Autodesk Inventor part; units mm, degrees
ref_plane "YZ Plane" through (0, 0, 0) normal (1, 0, 0) x (0, 1, 0)
ref_plane "XZ Plane" through (0, 0, 0) normal (0, 1, 0) x (-1, 0, 0)
ref_plane "XY Plane" through (0, 0, 0) normal (0, 0, 1) x (1, 0, 0)
sketch "Sketch1" plane through (0, 0, 0) normal (0, 1, 0) x (-1, 0, 0)
  line L0 (9.6232, 12.9345) -> (-6.3768, 12.9345)
  line L1 (-6.3768, 12.9345) -> (-6.3768, -20.0655)
  line L2 (-6.3768, -20.0655) -> (9.6232, -20.0655)
  line L3 (9.6232, -20.0655) -> (9.6232, 12.9345)
  dimension "d3" = 16
  dimension "d4" = 33
extrude "Extrusion1" add sketch "Sketch1" along normal blind 3
sketch "Sketch2" plane through (0, 3, 0) normal (0, 1, 0) x (1, 0, 0)
  circle A0 centre (2.3768, -8.9345) radius 1.75
  circle A1 centre (2.3768, 16.0655) radius 1.75
  line L0 (6.3768, -12.9345) -> (6.3768, 20.0655)
  line L1 (-9.6232, -12.9345) -> (6.3768, -12.9345)
  line L2 (6.3768, 20.0655) -> (-9.6232, 20.0655)
  point P0 (0, 0)
  dimension "d7" = 3.5
  dimension "d8" = 3.5
  dimension "d9" = 4
  dimension "d10" = 4
  dimension "d11" = 4
  dimension "d12" = 4
extrude "Extrusion2" cut sketch "Sketch2" against normal through all
ref_plane "Work Plane1" through (-9.6232, 0, -3.5655) normal (0, 0, 1) x (1, 0, 0)
sketch "Sketch4" plane through (-9.6232, 0, -3.5655) normal (0, 0, 1) x (1, 0, 0)
  line L0 (0, 0) -> (0, 3)
  circle A0 centre (0, 0) radius 3
  point P0 (9.6232, 0)
  dimension "d17" = 6
extrude "Extrusion3" add sketch "Sketch4" along normal mid plane 10
sketch "Sketch5" plane through (-9.6232, 0, 12.9345) normal (0, 0, 1) x (1, 0, 0)
  line L0 (0, 3) -> (0, 0)
  line L1 (3, -3) -> (-3, -3)
  line L2 (-3, -3) -> (-3, 3)
  line L3 (-3, 3) -> (3, 3)
  line L4 (3, 3) -> (3, -3)
  point P0 (9.6232, 0)
  point P1 (0, 2.5)
extrude "Extrusion4" cut sketch "Sketch5" against normal blind 11.5
mirror "Mirror1" about plane through (-9.6232, 0, -3.5655) normal (0, 0, 1) of "Extrusion4"
sketch "Sketch6" plane through (-9.6232, 0, 1.4345) normal (0, 0, 1) x (1, 0, 0)
  circle A0 centre (0, 0) radius 1.75
  point P0 (9.6232, 0)
  dimension "d24" = 3.5
extrude "Extrusion5" cut sketch "Sketch6" against normal up to next
sketch "Sketch7" plane through (0, 0, 0) normal (0, -1, 0) x (1, 0, 0)
  circle A0 centre (-3.6232, -16.0655) radius 2.75
  circle A1 centre (-3.6232, 8.9345) radius 2.75
  line L0 (6.3768, -20.0655) -> (-6.6232, -20.0655)
  line L1 (-6.6232, 12.9345) -> (6.3768, 12.9345)
  line L2 (-6.6232, 12.9345) -> (-6.6232, 1.4345)
  point P0 (0, 0)
  point P1 (-6.6232, 1.4345)
  dimension "d27" = 5.5
  dimension "d28" = 5.5
  dimension "d29" = 4
  dimension "d30" = 4
  dimension "d31" = 3
  dimension "d32" = 3
extrude "Extrusion6" cut sketch "Sketch7" against normal through all
equation "\"d11\" = d9"
equation "\"d12\" = d10"
equation "\"d30\" = d29"
equation "\"d32\" = d31"
properties part number "k2_hinge1_top"
Geometry check sheet. Reference: the model listing, model coordinates, mm. A direction names the side the tool comes from. Give positions to 0.01 mm unless a question says otherwise; leave off trailing zeros. Write each loop counter-clockwise with the first axis right and the second up, starting at its lowest first coordinate (ties: lowest second). Pieces come first, ordered by that corner, then holes.
1) Gauge pin test, flat ends, axial feed: pin 1 (1 mm diameter, centred on x = -7, z = -4.5, fed in from -Y); pin 2 (1.5 mm diameter, centred on y = 1, z = -12.5, fed in from -X); pin 3 (3.5 mm diameter, centred on x = -3.62, z = -16.07, fed in from -Y); pin 4 (3 mm diameter, centred on x = -11, y = 1, fed in from -Z). Record the tip position at first contact, or that the pin passes through.
2) Section check C-C, the plane z = -1. Record the boundary of the cut face in (x, y).
3) Material ranges on L1, parallel to X at y = 1.25, z = 9; L2, parallel to Z at x = 2.5, y = 1.4; L3, parallel to X at y = 2.15, z = 9.5, recorded low to high.
4) Section check A-A, the plane z = 10. Record the boundary of the cut face in (x, y), and give its area (3 significant figures).
5) Release check for a two-part mould opening along X. For faces 4 (the flat face through (-8, 1, 1.434)), 5 (the cylindrical face through (-10.913, 1.183, -3.496)), 6 (the flat face through (-6.623, 2, 7)) record: pulls with the +X half, pulls with the -X half, needs draft (parallel to the pull), parting line crosses it, or undercut.
6) Access from +Z, -Z, +X, -X, +Y, -Y to the whole of each face (thin tool, end or side, straight path). Record for faces 1 (the cylindrical face through (-2.14, 1.48, -13.75)), 2 (the flat face through (-8, 1, -8.566)), 3 (the flat face through (0, 0, -3)).
7) Section check D-D, the plane x = -9. Record the boundary of the cut face in (y, z).
8) Section check B-B, the plane x = -5.25. Record the boundary of the cut face in (y, z).
Computed:
1. pin 1: stops at y = -2.12
1. pin 2: stops at x = -6.62
1. pin 3: passes through
1. pin 4: stops at z = -8.57
2. outline: (-9.62, 3) arc R3 ccw (long way) to (-6.62, 0) - (6.38, 0) - (6.38, 3) - close; hole circle Ø3.5 at (-9.62, 0)
3. L1: x = -6.62 to -6.37, -0.87 to 0.63, 4.13 to 6.38
3. L2: z = -20.07 to -17.81, -14.32 to 7.19, 10.68 to 12.93
3. L3: x = -6.62 to -6.31, -0.93 to 0.72, 4.03 to 6.38
4. outline: (-6.62, 0) - (-6.16, 0) - (-6.16, 3) - (-6.62, 3) - close; (-1.09, 0) - (0.99, 0) - (0.99, 3) - (-1.09, 3) - close; (3.77, 0) - (6.38, 0) - (6.38, 3) - (3.77, 3) - close
4. area: 15.5 mm2
5. face 4: needs draft
5. face 5: undercut
5. face 6: pulls with the -X half
6. face 1: +Y, -Y
6. face 2: -Z, -X, +Y, -Y
6. face 3: +Z, -Z, +X, -Y
7. outline: (-2.93, -8.57) - (-1.64, -8.57) - (-1.64, 1.43) - (-2.93, 1.43) - close; (1.64, -8.57) - (3, -8.57) - (3, 1.43) - (1.64, 1.43) - close
8. outline: (0, -20.07) - (3, -20.07) - (3, -18.28) - (0, -18.28) - close; (0, -13.85) - (3, -13.85) - (3, 6.72) - (0, 6.72) - close; (0, 11.15) - (3, 11.15) - (3, 12.93) - (0, 12.93) - close
